CAD build for the part. Positions are in the model's coordinates, mm. A direction names the side the tool comes from. Round coordinates to 2 decimals unless told otherwise and drop trailing zeros. Write each loop counter-clockwise with the first axis right and the second up, starting at its lowest first coordinate (ties: lowest second). Pieces come first, ordered by that corner, then holes. Notation, with made-up numbers: M 42.5,87.5 L 91.5,87.5 A25 ccw 91.5,113.5 Z; hole C -7.75,60.5 d10. An arc over 180 degrees is marked long. Write each question's results on one line, items separated by ' | '. Start each with the question number.
```python
from build123d import *

# Parameters (mm, degrees)
BOSS_EXTRUDE1_DEPTH = 18.5
SKETCH2_W           = 6.45
SKETCH2_H           = 3.3
CUT_EXTRUDE1_DEPTH  = 4.5
SKETCH3_R           = 2.25
CUT_EXTRUDE2_DEPTH  = 1.75
SKETCH4_R           = 1.15
CUT_EXTRUDE3_DEPTH  = 2.3
FILLET3_R           = 2
FILLET4_R           = 2
FILLET5_R           = 2
FILLET6_R           = 2
FILLET7_R           = 1
FILLET8_R           = 0.5
FILLET9_R           = 1
FILLET10_R          = 1
FILLET12_R          = 0.5


with BuildPart() as part:
    # Sketch1 → Boss-Extrude1 (new body)
    with BuildSketch(Plane(origin=(0, 0, 0), x_dir=(1, 0, 0), z_dir=(0, 1, 0))):
        Polygon((0, 0), (0, 11.227239651), (4, 11.227239651), (4, 4.427239651), (22.45, 4.427239651), (22.45, 0), align=None)
    extrude(amount=BOSS_EXTRUDE1_DEPTH)

    # Sketch2 → Cut-Extrude1 (cut)
    with BuildSketch(Plane.XY):
        with Locations((11.225, 9.25)):
            Rectangle(SKETCH2_W, SKETCH2_H)
    extrude(amount=-CUT_EXTRUDE1_DEPTH, mode=Mode.SUBTRACT)

    # Sketch3 → Cut-Extrude2 (cut)
    with BuildSketch(Plane(origin=(4, 0, 0), x_dir=(0, 0, -1), z_dir=(1, 0, 0))):
        with Locations((7.827239651, 9.25)):
            Circle(SKETCH3_R)
    extrude(amount=-CUT_EXTRUDE2_DEPTH, mode=Mode.SUBTRACT)

    # Sketch4 → Cut-Extrude3 (cut)
    with BuildSketch(Plane(origin=(2.25, 0, 0), x_dir=(0, 0, -1), z_dir=(1, 0, 0))):
        with Locations((7.827239651, 9.25)):
            Circle(SKETCH4_R)
    extrude(amount=-CUT_EXTRUDE3_DEPTH, mode=Mode.SUBTRACT)

    # Fillet3
    fillet3_edges = [part.edges().sort_by_distance(p)[0] for p in [
        (2, 18.5, -11.227239651),
    ]]
    fillet(fillet3_edges, radius=FILLET3_R)

    # Fillet4
    fillet4_edges = [part.edges().sort_by_distance(p)[0] for p in [
        (2, 0, -11.227239651),
    ]]
    fillet(fillet4_edges, radius=FILLET4_R)

    # Fillet5
    fillet5_edges = [part.edges().sort_by_distance(p)[0] for p in [
        (22.45, 0, -2.213619825),
    ]]
    fillet(fillet5_edges, radius=FILLET5_R)

    # Fillet6
    fillet6_edges = [part.edges().sort_by_distance(p)[0] for p in [
        (22.45, 18.5, -2.213619825),
    ]]
    fillet(fillet6_edges, radius=FILLET6_R)

    # Fillet7
    fillet7_edges = [part.edges().sort_by_distance(p)[0] for p in [
        (11.225, 10.9, -4.427239651),
        (8, 9.25, -4.427239651),
        (11.225, 7.6, -4.427239651),
        (14.45, 9.25, -4.427239651),
    ]]
    fillet(fillet7_edges, radius=FILLET7_R)

    # Fillet8
    fillet8_edges = [part.edges().sort_by_distance(p)[0] for p in [
        (4, 9.25, -5.577239651),
    ]]
    fillet(fillet8_edges, radius=FILLET8_R)

    # Fillet9
    fillet9_edges = [part.edges().sort_by_distance(p)[0] for p in [
        (2.25, 9.25, -5.577239651),
    ]]
    fillet(fillet9_edges, radius=FILLET9_R)

    # Fillet10
    fillet10_edges = [part.edges().sort_by_distance(p)[0] for p in [
        (12.225, 0, -4.427239651),
        (21.864213562, 0.585786438, -4.427239651),
        (12.225, 18.5, -4.427239651),
        (22.45, 9.25, -4.427239651),
        (21.864213562, 17.914213562, -4.427239651),
    ]]
    fillet(fillet10_edges, radius=FILLET10_R)

    # Fillet12
    fillet12_edges = [part.edges().sort_by_distance(p)[0] for p in [
        (4, 18.5, -6.827239651),
        (4, 9.25, -11.227239651),
        (4, 17.914213562, -10.641453213),
        (4, 0.585786438, -10.641453213),
        (4, 0, -6.827239651),
    ]]
    fillet(fillet12_edges, radius=FILLET12_R)


solid = part.part
```
1) Wall check: line 1 along X through (y, z) = (6, -8.75); line 2 along Z through (x, y) = (17, 8); line 3 along Y through (x, z) = (2, -7). Give the ranges that are in metal, low to high. Write a range as from..to.
2) Saw through at D-D, the plane x = 16. Write the cut outline in (y, z), plus the area to 3 significant figures.
3) Pull direction X, two halves, no side cores. Call faces 1 (the face through (1.141, 8.127, -7.578)), 2 (the face through (11, 7.6, -2)), 3 (the face through (21.85, 0.57, -1.69)): pulls with the +X half, pulls with the -X half, needs draft (parallel to the pull), parting line crosses it, or undercut.
4) Saw through at B-B, the plane y = 9.25. Write the cut outline in (x, z), plus the area to 3 significant figures.
5) Saw through at C-C, the plane z = -2.5. Write the cut outline in (x, y), plus the area to 3 significant figures.
6) Drop flat-ended pins along their axis: pin 1 Ø6 at (y, z) = (9.25, -7.83) entering from +X; pin 2 Ø1.5 at (y, z) = (2, -5) entering from +X; pin 3 Ø8 at (x, y) = (15.5, 8.5) entering from -Z; pin 4 Ø0.7 at (y, z) = (9.5, -8.5) entering from +X. Give the stop position or say it passes through.
7) Saw through at A-A, the plane x = 12. Write the cut outline in (y, z).
8) 3-axis set-ups, long thin cutter, end or side, ignore diameter. For faces 4 (the face through (8, 9, -2)), 5 (the face through (11.17, 7.31, -4.13)), 6 (the face through (21.88, 17.9, -1.69)), 7 (the face through (4, 9.1, -4.7)), 8 (the face through (11.86, 18.21, -4.13)): which of +Z, -Z, +X, -X, +Y, -Y reach the whole face in a straight line?
Filled sheet:
1) line 1: x = 0..4 | line 2: z = -4.43..0 | line 3: y = 0..8.45, 10.05..18.5
2) outline: M 0,-3.43 A1 ccw 1,-4.43 L 17.5,-4.43 A1 ccw 18.5,-3.43 L 18.5,0 L 0,0 Z | area: 81.5 mm^2
3) face 1: needs draft | face 2: undercut | face 3: pulls with the +X half
4) outline: M 0,-11.23 L 3.5,-11.23 A0.5 ccw 4,-10.73 L 4,-10.58 A0.5 ccw 3.5,-10.08 L 3.25,-10.08 A1 cw 2.25,-9.08 L 2.25,-8.98 L 0,-8.98 Z; M 0,-6.68 L 2.25,-6.68 L 2.25,-6.58 A1 cw 3.25,-5.58 L 3.5,-5.58 A0.5 ccw 4,-5.08 L 4,-4.43 L 7,-4.43 A1 ccw 8,-3.43 L 8,0 L 0,0 Z; M 14.45,-3.43 A1 ccw 15.45,-4.43 L 21.45,-4.43 A1 ccw 22.45,-3.43 L 22.45,0 L 14.45,0 Z | area: 84.6 mm^2
5) outline: M 0,0 L 20.45,0 A2 ccw 22.45,2 L 22.45,16.5 A2 ccw 20.45,18.5 L 0,18.5 Z; hole M 8,7.6 L 14.45,7.6 L 14.45,10.9 L 8,10.9 Z | area: 392 mm^2
6) pin 1: stops at x = 4 | pin 2: stops at x = 22.02 | pin 3: stops at z = -4.43 | pin 4: passes through
7) outline: M 0,-3.43 A1 ccw 1,-4.43 L 6.6,-4.43 A1 ccw 7.6,-3.43 L 7.6,0 L 0,0 Z; M 10.9,-3.43 A1 ccw 11.9,-4.43 L 17.5,-4.43 A1 ccw 18.5,-3.43 L 18.5,0 L 10.9,0 Z
8) face 4: +Z, -Z | face 5: -Z | face 6: +Z, -Z, +X, +Y | face 7: -Z, +X, +Y, -Y | face 8: -Z, +X, +Y
